from build123d import *

# Parameters (mm, degrees)
F0_R             = 6.35
F1_DEPTH         = 12.7
F3_DEPTH         = 38.1
F7_DEPTH         = 89.8035612107
F8_R             = 2.54
F9_DEPTH         = 6.35
F9_COPIES_COUNT  = 2
F9_COPIES_PITCH  = 14.929745
F9_COPIES1_COUNT = 2
F9_COPIES1_PITCH = 14.929745
F9_COPIES2_COUNT = 2
F9_COPIES2_PITCH = 24.156836
F9_COPIES3_COUNT = 2
F9_COPIES3_PITCH = 24.156836


# Not quite as in the source:
# - a pattern or mirror of a feature is missing from the dataset's text; its kind, count and spacing are read off the source's solid


with BuildPart() as f1:
    # F0 (on Top) → F1 (new body)
    with BuildSketch(Plane.XY):
        with BuildLine():
            Line((12.7, 50.8), (12.7, 63.5))
            ThreePointArc((12.7, 63.5), (0, 76.2), (-12.7, 63.5))
            Line((-12.7, 63.5), (-12.7, 38.1))
            Line((-12.7, 38.1), (0, 38.1))
            ThreePointArc((0, 38.1), (6.35, 31.75), (0, 25.4))
            Line((0, 25.4), (-12.7, 25.4))
            Line((-12.7, 25.4), (-12.7, 0))
            ThreePointArc((-12.7, 0), (0, -12.7), (12.7, 0))
            Line((12.7, 0), (12.7, 12.7))
            Line((12.7, 12.7), (76.2, 12.7))
            Line((76.2, 12.7), (76.2, 0))
            ThreePointArc((76.2, 0), (88.9, -12.7), (101.6, 0))
            Line((101.6, 0), (101.6, 63.5))
            ThreePointArc((101.6, 63.5), (88.9, 76.2), (76.2, 63.5))
            Line((76.2, 63.5), (76.2, 50.8))
            Line((76.2, 50.8), (12.7, 50.8))
        make_face()
        Circle(F0_R, mode=Mode.SUBTRACT)
        with Locations((88.9, 0)):
            Circle(F0_R, mode=Mode.SUBTRACT)
        with Locations((0, 63.5)):
            Circle(F0_R, mode=Mode.SUBTRACT)
        with Locations((88.9, 63.5)):
            Circle(F0_R, mode=Mode.SUBTRACT)
    extrude(amount=F1_DEPTH)

    # F2 (on face) → F3 (join)
    with BuildSketch(Plane.XZ.offset(-12.7)):
        Polygon((76.2, 12.7), (101.6, 12.7), (76.9042956671, 37.3957043329), (52.2085913341, 12.7), align=None)
    extrude(amount=-F3_DEPTH)

    # F4 (on face) → F5 (join, up to the next surface of F1)
    with BuildSketch(Plane(origin=(57.15, 0, 57.15), x_dir=(0.7071067812, 0, -0.7071067812), z_dir=(0.7071067812, 0, 0.7071067812))):
        with BuildLine():
            ThreePointArc((27.9367928475, 24.13), (20.3167928475, 31.75), (27.9367928475, 39.37))
            Line((27.9367928475, 39.37), (27.9367928475, 50.8))
            ThreePointArc((27.9367928475, 50.8), (8.8867928475, 31.75), (27.9367928475, 12.7))
            Line((27.9367928475, 12.7), (27.9367928475, 24.13))
        make_face()
    extrude(until=Until.NEXT, dir=(-0.7071067812, 0, -0.7071067812))

    # F6 (on face) → F7 (cut, through all)
    with BuildSketch(Plane(origin=(57.15, 0, 57.15), x_dir=(0.7071067812, 0, -0.7071067812), z_dir=(0.7071067812, 0, 0.7071067812))):
        with BuildLine():
            ThreePointArc((27.9367928475, 24.13), (33.3249465201, 26.3618463274), (35.5567928475, 31.75))
            ThreePointArc((35.5567928475, 31.75), (33.3249465201, 37.1381536726), (27.9367928475, 39.37))
            Line((27.9367928475, 39.37), (27.9367928475, 24.13))
        make_face()
        with BuildLine():
            Line((27.9367928475, 24.13), (27.9367928475, 39.37))
            ThreePointArc((27.9367928475, 39.37), (20.3167928475, 31.75), (27.9367928475, 24.13))
        make_face()
    extrude(amount=-F7_DEPTH, mode=Mode.SUBTRACT)

    # F8 (on face) → F9 (cut)
    with BuildSketch(Plane(origin=(57.15, 0, 57.15), x_dir=(0.7071067812, 0, -0.7071067812), z_dir=(0.7071067812, 0, 0.7071067812))):
        with Locations((15.2367928475, 31.75)):
            Circle(F8_R)
    f9 = extrude(amount=-F9_DEPTH, mode=Mode.SUBTRACT)

    # F9_copies: F9 ×2
    with Locations(*[Vector(0.4156269378, 0.8090169944, -0.4156269378) * (i * F9_COPIES_PITCH) for i in range(1, F9_COPIES_COUNT)]):
        add(f9, mode=Mode.SUBTRACT)

    # F9_copies1: F9 ×2
    with Locations(*[Vector(0.4156269378, -0.8090169944, -0.4156269378) * (i * F9_COPIES1_PITCH) for i in range(1, F9_COPIES1_COUNT)]):
        add(f9, mode=Mode.SUBTRACT)

    # F9_copies2: F9 ×2
    with Locations(*[Vector(0.672498512, -0.3090169944, -0.672498512) * (i * F9_COPIES2_PITCH) for i in range(1, F9_COPIES2_COUNT)]):
        add(f9, mode=Mode.SUBTRACT)

    # F9_copies3: F9 ×2
    with Locations(*[Vector(0.672498512, 0.3090169944, -0.672498512) * (i * F9_COPIES3_PITCH) for i in range(1, F9_COPIES3_COUNT)]):
        add(f9, mode=Mode.SUBTRACT)


solid = f1.part
Source: CAD feature listing. Evaluate the final solid. Frame: model axes, mm. A direction names the side the tool comes from. Coordinates: 2 decimals unless noted, no trailing zeros. Loops run counter-clockwise (first coordinate to the right, second up) from the corner with the lowest first, then second, coordinate; pieces in that order, holes last. Notation, with made-up numbers: (2.5, 47) - (31.5, 47) arc R18 cw to (31.5, 74) - close; hole circle Ø7 at (38.25, -5). An arc over 180 degrees is marked (long way). One line per item, written item: value. Start each with the question number.
1. Section B-B (y = 55.5). Return the cut outline in (x, z), and give its area (3 significant figures).
2. Section D-D (z = 9). State how many separate pieces and enclosed holes the cut face has, and give its area (3 significant figures).
3. Set-up query: faces 1 (the flat face through (79.65, 39.25, 25.67)), 2 (the flat face through (76.2, 57, 6)), 3 (the flat face through (89, 55, 12.7)), 4 (the flat face through (12.7, 6, 6)). Return all of +Z, -Z, +X, -X, +Y, -Y with unobstructed straight access to the full face (end or side cutting, diameter ignored); none if empty.
4. Mould query, pull axis X, two halves, no side actions, for faces 5 (the flat face through (69.61, 19.71, 35.71)), 6 (the flat face through (57, 50.8, 15)), 7 (the flat face through (-6, 38.1, 6)), 8 (the flat face through (101.6, 31, 6)). Classes: pulls with the +X half, pulls with the -X half, needs draft (parallel to the pull), parting line crosses it, or undercut.
5. Section A-A (x = 88.9). Return the cut outline in (y, z), and give its area (3 significant figures).
6. Contact query for flat-ended pins moving along their axis: P1, Ø4, axis at x = -9, z = 8.5, coming from the -Y side; P2, Ø6.5, axis at x = -4.5, z = 6.5, coming from the +Y side; P3, Ø7.5, axis at x = 88.9, y = 0, coming from the +Z side; P4, Ø3, axis at x = 50, y = 48.5, coming from the -Z side. Output: stop coordinate, or through.
7. Section C-C (y = -5). Return the cut outline in (x, z).
8. Ray query, L1, parallel to Y at x = 88.9, z = 4.5; L2, parallel to X at y = 63, z = 4; L3, parallel to X at y = 8, z = 12. Return the intervals inside material, ascending.
Verdict:
1. outline: (-12.7, 0) - (12.7, 0) - (12.7, 12.7) - (-12.7, 12.7) - close; (76.2, 0) - (101.6, 0) - (101.6, 12.7) - (76.2, 12.7) - close
1. area: 645 mm2
2. separate pieces: 1
2. enclosed holes: 5
2. area: 5,670 mm2
3. face 1: none
3. face 2: +Z, -Z, +Y
3. face 3: +Z, +X, -X, +Y
3. face 4: +Z, -Z, -Y
4. face 5: undercut
4. face 6: undercut
4. face 7: needs draft
4. face 8: pulls with the +X half
5. outline: (-12.7, 0) - (-6.35, 0) - (-6.35, 12.7) - (-12.7, 12.7) - close; (6.35, 0) - (57.15, 0) - (57.15, 12.7) - (50.8, 12.7) - (50.8, 25.4) - (12.7, 25.4) - (12.7, 12.7) - (6.35, 12.7) - close; (69.85, 0) - (76.2, 0) - (76.2, 12.7) - (69.85, 12.7) - close
5. area: 1,290 mm2
6. P1: stops at y = -10.6
6. P2: stops at y = 76.14
6. P3: passes through
6. P4: stops at z = 0
7. outline: (-11.67, 0) - (-3.91, 0) - (-3.91, 12.7) - (-11.67, 12.7) - close; (3.91, 0) - (11.67, 0) - (11.67, 12.7) - (3.91, 12.7) - close; (77.23, 0) - (84.99, 0) - (84.99, 12.7) - (77.23, 12.7) - close; (92.81, 0) - (100.57, 0) - (100.57, 12.7) - (92.81, 12.7) - close
8. L1: y = -12.7 to -6.35, 6.35 to 57.15, 69.85 to 76.2
8. L2: x = -12.7 to -6.33, 6.33 to 12.7, 76.2 to 82.57, 95.23 to 101.6
8. L3: x = -12.7 to 12.7, 76.2 to 101.6
